Here's how the part is built. I have some questions about the finished solid (model axes, mm). A direction names the side the tool comes from. Coordinates: 2 decimals unless noted, no trailing zeros. Write each loop counter-clockwise with the first axis right and the second up, starting at its lowest first coordinate (ties: lowest second). Pieces come first, ordered by that corner, then holes. Notation, with made-up numbers: (-32, -17) -> (9, -17) arc R25 ccw to (9, -3) -> close; hole circle Ø4 at (24, 66.5). An arc over 180 degrees is marked (long way). Answer in a Markdown table with one row per item. Add a question column.
from build123d import *

# Parameters (mm, degrees)
BOSS_EXTRUDE1_DEPTH = 6.35
SKETCH6_R           = 4.250000001
CUT_EXTRUDE1_DEPTH  = 7.35
SKETCH2_W           = 6.85
SKETCH2_H           = 6.85
BOSS_EXTRUDE2_DEPTH = 25.4
SKETCH7_W           = 6.35
SKETCH7_H           = 4
BOSS_EXTRUDE3_DEPTH = 6.35
SKETCH9_R           = 2
CUT_EXTRUDE2_DEPTH  = 6.540000128
CIRPATTERN1_COUNT   = 3
SKETCH10_R          = 1.7145
CUT_EXTRUDE3_DEPTH  = 2
CIRPATTERN2_COUNT   = 3
CUT_EXTRUDE4_DEPTH  = 6.35
FILLET1_R           = 2.54
SKETCH12_R          = 7.5
SKETCH12_R_2        = 4.250000001
BOSS_EXTRUDE4_DEPTH = 6


with BuildPart() as part:
    # Sketch1 → Boss-Extrude1 (new body)
    with BuildSketch(Plane(origin=(0, 0, 0), x_dir=(1, 0, 0), z_dir=(0, 1, 0))):
        Polygon((19.05, -32.995567884), (38.1, 0), (19.05, 32.995567884), (-19.05, 32.995567884), (-38.1, 0), (-19.05, -32.995567884), align=None)
    extrude(amount=BOSS_EXTRUDE1_DEPTH)

    # Sketch6 → Cut-Extrude1 (cut, through all)
    with BuildSketch(Plane(origin=(0, 6.35, 0), x_dir=(1, 0, 0), z_dir=(0, 1, 0))):
        Circle(SKETCH6_R)
    extrude(amount=-CUT_EXTRUDE1_DEPTH, mode=Mode.SUBTRACT)

    # Sketch2 → Boss-Extrude2 (add)
    with BuildSketch(Plane.XZ):
        with BuildLine():
            Line((-5.425, 15.1), (-5.425, 4.25))
            Line((-5.425, 4.25), (-2.067021045, 4.25))
            ThreePointArc((-2.067021045, 4.25), (0, 4.726), (2.067021045, 4.25))
            Line((2.067021045, 4.25), (5.425, 4.25))
            Line((5.425, 4.25), (5.425, 15.1))
            Line((5.425, 15.1), (-5.425, 15.1))
        make_face()
        with Locations((0, 9.675)):
            Rectangle(SKETCH2_W, SKETCH2_H, mode=Mode.SUBTRACT)
        with BuildLine():
            Line((2.647097444, -3.915092735), (0.968107966, -6.823187816))
            Line((0.968107966, -6.823187816), (10.364483597, -12.248187816))
            Line((10.364483597, -12.248187816), (15.789483597, -2.851812184))
            Line((15.789483597, -2.851812184), (6.393107966, 2.573187816))
            Line((6.393107966, 2.573187816), (4.714118489, -0.334907265))
            ThreePointArc((4.714118489, -0.334907265), (4.092836058, -2.363), (2.647097444, -3.915092735))
        make_face()
        Polygon((13.05743279, -3.583862992), (7.125158774, -0.158862992), (3.700158774, -6.091137008), (9.63243279, -9.516137008), align=None, mode=Mode.SUBTRACT)
        with BuildLine():
            Line((-4.714118489, -0.334907265), (-6.393107966, 2.573187816))
            Line((-6.393107966, 2.573187816), (-15.789483597, -2.851812184))
            Line((-15.789483597, -2.851812184), (-10.364483597, -12.248187816))
            Line((-10.364483597, -12.248187816), (-0.968107966, -6.823187816))
            Line((-0.968107966, -6.823187816), (-2.647097444, -3.915092735))
            ThreePointArc((-2.647097444, -3.915092735), (-4.092836058, -2.363), (-4.714118489, -0.334907265))
        make_face()
        Polygon((-9.63243279, -9.516137008), (-3.700158774, -6.091137008), (-7.125158774, -0.158862992), (-13.05743279, -3.583862992), align=None, mode=Mode.SUBTRACT)
    extrude(amount=BOSS_EXTRUDE2_DEPTH)

    # Sketch7 → Boss-Extrude3 (add)
    with BuildSketch(Plane.XZ):
        with Locations((-11.640300372, 20.97230006)):
            Rectangle(SKETCH7_W, SKETCH7_H)
        with Locations((-11.640300372, 29.97230006)):
            Rectangle(SKETCH7_W, SKETCH7_H)
        Polygon((27.296626747, 1.354008633), (24.121626747, -4.145252681), (20.657525132, -2.145252681), (23.832525132, 3.354008633), align=None)
        Polygon((31.626753766, -1.145991367), (35.090855381, -3.145991367), (31.915855381, -8.645252681), (28.451753766, -6.645252681), align=None)
        Polygon((-12.481326375, -24.306844341), (-15.656326375, -18.807583027), (-12.19222476, -16.807583027), (-9.01722476, -22.306844341), align=None)
        Polygon((-16.811453394, -26.806844341), (-20.275555009, -28.806844341), (-23.450555009, -23.307583027), (-19.986453394, -21.307583027), align=None)
    extrude(amount=BOSS_EXTRUDE3_DEPTH)

    # Sketch9 → Cut-Extrude2 (cut)
    with BuildSketch(Plane.XY.offset(31.97230006)):
        with Locations((-11.640300372, -3.262620176)):
            Circle(SKETCH9_R)
    cut_extrude2 = extrude(amount=-CUT_EXTRUDE2_DEPTH, mode=Mode.SUBTRACT)

    # CirPattern1: Cut-Extrude2 ×3 about axis
    cirpattern1_axis = Axis((0, 0, 0), (0, 1, 0))
    for i in range(1, CIRPATTERN1_COUNT):
        add(cut_extrude2.rotate(cirpattern1_axis, i * 360 / CIRPATTERN1_COUNT), mode=Mode.SUBTRACT)

    # Sketch10 → Cut-Extrude3 (cut)
    with BuildSketch(Plane.XY.offset(22.97230006)):
        with Locations((-11.640300372, -3.262620176)):
            Circle(SKETCH10_R)
    cut_extrude3 = extrude(amount=-CUT_EXTRUDE3_DEPTH, mode=Mode.SUBTRACT)

    # CirPattern2: Cut-Extrude3 ×3 about axis
    cirpattern2_axis = Axis((0, 0, 0), (0, 1, 0))
    for i in range(1, CIRPATTERN2_COUNT):
        add(cut_extrude3.rotate(cirpattern2_axis, i * 360 / CIRPATTERN2_COUNT), mode=Mode.SUBTRACT)

    # Sketch11 → Cut-Extrude4 (cut)
    with BuildSketch(Plane.XZ):
        Polygon((-38.1, 0), (-19.05, 32.995567884), (-20.416871812, -0.535432071), (-12.999443709, -13.382794406), (-26.285912957, -20.462599003), align=None)
        Polygon((19.05, 32.995567884), (38.1, 0), (9.74473813, 17.94924569), (-5.090118075, 17.94924569), (-4.578174086, 32.995567884), align=None)
        Polygon((19.05, -32.995567884), (-19.05, -32.995567884), (10.672133681, -17.413813619), (18.089561784, -4.566451284), (30.864087043, -12.532968881), align=None)
    extrude(amount=-CUT_EXTRUDE4_DEPTH, mode=Mode.SUBTRACT)

    # Fillet1
    fillet1_edges = [part.edges().sort_by_distance(p)[0] for p in [
        (38.1, 3.175, 0),
        (-19.05, 3.175, 32.995567884),
        (-19.05, 3.175, -32.995567884),
        (18.089561784, 3.175, -4.566451284),
        (10.672133681, 3.175, -17.413813619),
        (30.864087043, 3.175, -12.532968881),
        (-5.090118075, 3.175, 17.94924569),
        (9.74473813, 3.175, 17.94924569),
        (-4.578174086, 3.175, 32.995567884),
        (-12.999443709, 3.175, -13.382794406),
        (-20.416871812, 3.175, -0.535432071),
        (-26.285912957, 3.175, -20.462599003),
    ]]
    fillet(fillet1_edges, radius=FILLET1_R)

    # Sketch12 → Boss-Extrude4 (add)
    with BuildSketch(Plane(origin=(0, 6.35, 0), x_dir=(1, 0, 0), z_dir=(0, 1, 0))):
        Circle(SKETCH12_R)
        Circle(SKETCH12_R_2, mode=Mode.SUBTRACT)
    extrude(amount=BOSS_EXTRUDE4_DEPTH)


solid = part.part
Q1. Imagine slicing it at B-B on x = 0. Please give me the cut outline in (y, z).
Q2. I need wall thicknesses on line 1 (Z direction, x = -4, y = -14); line 2 (X direction, y = -1, z = -6); line 3 (X direction, y = -14.5, z = 9) (3 decimals). Which ranges of each line are inside material? Lowest first, please. Write a range as [from, to].
Q3. I'm going to push flat-ended pins straight in: P1, Ø7.5, axis at x = -1.5, y = -6.5, coming from the +Z side; P2, Ø6, axis at y = -11, z = 21.5, coming from the -X side; P3, Ø4, axis at x = -11, y = -3, coming from the +Z side; P4, Ø7, axis at x = 2.5, y = 3.5, coming from the +Z side. Where does each tip first touch, or does it pass through?
Q4. For faces 1 (the cylindrical face through (-12.012, -4.936, 21.986)), 2 (the flat face through (4, -13, 4.25)), 3 (the flat face through (-12, -6.35, 30)), 4 (the flat face through (-11.026, -12.522, -0.101)), which set-ups out of +Z, -Z, +X, -X, +Y, -Y let a thin tool reach every point of the face, with its end or its side?
Q5. Imagine slicing it at A-A on y = -12. State how many separate pieces and enclosed holes the cut face has, plus the area to 3 significant figures.
Q6. If we mould it in two halves opening along Z, with no side actions, what happens to faces 5 (the cylindrical face through (-0.03, -12.522, 4.726)), 6 (the cylindrical face through (-25.206, 3.219, -20.742)), 7 (the cylindrical face through (-18.803, 3.219, -32.046))? For each: pulls with the +Z half, pulls with the -Z half, needs draft (parallel to the pull), parting line crosses it, or undercut.
Result sheet:
| question | item | result |
|---|---|---|
| 1 | outline | (-25.4, 4.73) -> (0, 4.73) -> (0, 4.25) -> (12.35, 4.25) -> (12.35, 7.5) -> (6.35, 7.5) -> (6.35, 17.95) -> (0, 17.95) -> (0, 15.1) -> (-25.4, 15.1) -> (-25.4, 13.1) -> (0, 13.1) -> (0, 6.25) -> (-25.4, 6.25) -> close; (0, -23.01) -> (6.35, -23.01) -> (6.35, -7.5) -> (12.35, -7.5) -> (12.35, -4.25) -> (0, -4.25) -> close |
| 2 | line 1 | z = [-8.57, -6.26], [-5.57, -2.52], [4.25, 15.1] |
| 2 | line 2 | x = [-13.97, -11.66], [-3.75, -1.44], [1.44, 3.75], [11.66, 13.97], [28.82, 33.44] |
| 2 | line 3 | x = [-5.425, -3.425], [3.425, 5.425] |
| 3 | P1 | stops at z = 15.1 |
| 3 | P2 | passes through |
| 3 | P3 | stops at z = 31.97 |
| 3 | P4 | stops at z = 17.95 |
| 4 | face 1 | +Z |
| 4 | face 2 | +X, -X, -Y |
| 4 | face 3 | +Z, +X, -X, -Y |
| 4 | face 4 | -X, -Y |
| 5 | separate pieces | 3 |
| 5 | enclosed holes | 3 |
| 5 | area | 208 mm^2 |
| 6 | face 5 | undercut |
| 6 | face 6 | parting line crosses it |
| 6 | face 7 | pulls with the -Z half |
